```python
from build123d import *

# Parameters (mm, degrees)
SKETCH1_W                          = 165.1
SKETCH1_H                          = 12.7
BOSS_EXTRUDE1_DEPTH                = 127
SKETCH2_R                          = 20.6375
CUT_EXTRUDE1_DEPTH                 = 153.002606886
CUT_EXTRUDE3_DEPTH                 = 153.002606886
FILLET1_R                          = 3.175
FILLET2_R                          = 1.5875
SKETCH5_W                          = 101.6
SKETCH5_H                          = 9.525
CUT_EXTRUDE4_DEPTH                 = 153.002606886
FILLET3_R                          = 3.175
F_1_16_0_0625_DIAMETER_HOLE1_D     = 1.5875
F_1_16_0_0625_DIAMETER_HOLE1_DEPTH = 15.875
F_1_16_0_0625_DIAMETER_HOLE1_TIP   = 0.476933116
F_1_16_0_0625_DIAMETER_HOLE2_D     = 1.5875
F_1_16_0_0625_DIAMETER_HOLE2_DEPTH = 15.875
F_1_16_0_0625_DIAMETER_HOLE2_TIP   = 0.476933116
CUT_EXTRUDE5_DEPTH                 = 153.002606886


with BuildPart() as part:
    # Sketch1 → Boss-Extrude1 (new, symmetric)
    with BuildSketch(Plane(origin=(0, 0, 0), x_dir=(1, 0, 0), z_dir=(0, 1, 0))):
        Rectangle(SKETCH1_W, SKETCH1_H)
    extrude(amount=BOSS_EXTRUDE1_DEPTH, both=True)

    # Sketch2 → Cut-Extrude1 (cut, through all)
    with BuildSketch(Plane.XY.offset(6.35)):
        with Locations((0, 127)):
            Circle(SKETCH2_R)
    extrude(amount=-CUT_EXTRUDE1_DEPTH, mode=Mode.SUBTRACT)

    # Sketch4 → Cut-Extrude3 (cut, through all)
    with BuildSketch(Plane.XY.offset(6.35)):
        with BuildLine():
            Line((57.277, 127), (57.277, 104.775))
            Line((57.277, 104.775), (43.877983689, 104.775))
            Line((43.877983689, 104.775), (38.415383769, 114.236500603))
            ThreePointArc((38.415383769, 114.236500603), (39.624000301, 118.747116057), (44.134615883, 117.5385))
            Line((44.134615883, 117.5385), (47.690804866, 111.379))
            Line((47.690804866, 111.379), (50.673, 111.379))
            Line((50.673, 111.379), (50.673, 127))
            Line((50.673, 127), (57.277, 127))
        make_face()
        with BuildLine():
            Line((-50.673, 127), (-57.277, 127))
            Line((-57.277, 127), (-57.277, 104.775))
            Line((-57.277, 104.775), (-43.877983689, 104.775))
            Line((-43.877983689, 104.775), (-38.415383769, 114.236500603))
            ThreePointArc((-38.415383769, 114.236500603), (-39.624000301, 118.747116057), (-44.134615883, 117.5385))
            Line((-44.134615883, 117.5385), (-47.690804866, 111.379))
            Line((-47.690804866, 111.379), (-50.673, 111.379))
            Line((-50.673, 111.379), (-50.673, 127))
        make_face()
    extrude(amount=-CUT_EXTRUDE3_DEPTH, mode=Mode.SUBTRACT)

    # Fillet1
    fillet1_edges = [part.edges().sort_by_distance(p)[0] for p in [
        (50.673, 127, 0),
        (57.277, 127, 0),
        (57.277, 104.775, 0),
        (43.877983689, 104.775, 0),
        (-43.877983689, 104.775, 0),
        (-57.277, 104.775, 0),
        (-57.277, 127, 0),
        (-50.673, 127, 0),
    ]]
    fillet(fillet1_edges, radius=FILLET1_R)

    # Fillet2
    fillet2_edges = [part.edges().sort_by_distance(p)[0] for p in [
        (47.690804866, 111.379, 0),
        (50.673, 111.379, 0),
        (-50.673, 111.379, 0),
        (-47.690804866, 111.379, 0),
    ]]
    fillet(fillet2_edges, radius=FILLET2_R)

    # Sketch5 → Cut-Extrude4 (cut, through all)
    with BuildSketch(Plane.XY.offset(6.35)):
        with Locations((0, -122.2375)):
            Rectangle(SKETCH5_W, SKETCH5_H)
    extrude(amount=-CUT_EXTRUDE4_DEPTH, mode=Mode.SUBTRACT)

    # Fillet3
    fillet3_edges = [part.edges().sort_by_distance(p)[0] for p in [
        (-50.8, -127, 0),
        (-50.8, -117.475, 0),
        (50.8, -117.475, 0),
        (50.8, -127, 0),
    ]]
    fillet(fillet3_edges, radius=FILLET3_R)

    # 1/16 (0.0625) Diameter Hole1
    with Locations(Plane(origin=(82.55, 0, 0), x_dir=(0, 0, -1), z_dir=(1, 0, 0))):
        with Locations((0, -120.65), (0, -95.25), (0, 44.45), (0, 69.85), (0, 120.65)):
            Hole(F_1_16_0_0625_DIAMETER_HOLE1_D / 2, depth=F_1_16_0_0625_DIAMETER_HOLE1_DEPTH)
            with Locations((0, 0, -(F_1_16_0_0625_DIAMETER_HOLE1_DEPTH + F_1_16_0_0625_DIAMETER_HOLE1_TIP / 2))):  # 118° drill point
                Cone(0, F_1_16_0_0625_DIAMETER_HOLE1_D / 2, F_1_16_0_0625_DIAMETER_HOLE1_TIP, mode=Mode.SUBTRACT)

    # 1/16 (0.0625) Diameter Hole2
    with Locations(Plane.ZY.offset(82.55)):
        with Locations((0, -120.65), (0, -95.25), (0, 44.45), (0, 69.85), (0, 120.65)):
            Hole(F_1_16_0_0625_DIAMETER_HOLE2_D / 2, depth=F_1_16_0_0625_DIAMETER_HOLE2_DEPTH)
            with Locations((0, 0, -(F_1_16_0_0625_DIAMETER_HOLE2_DEPTH + F_1_16_0_0625_DIAMETER_HOLE2_TIP / 2))):  # 118° drill point
                Cone(0, F_1_16_0_0625_DIAMETER_HOLE2_D / 2, F_1_16_0_0625_DIAMETER_HOLE2_TIP, mode=Mode.SUBTRACT)

    # Sketch10 → Cut-Extrude5 (cut, through all)
    with BuildSketch(Plane.XY.offset(6.35)):
        with BuildLine():
            Line((-61.89437725, -88.484920775), (-50.783316982, 38.515079225))
            ThreePointArc((-50.783316982, 38.515079225), (-45.623860507, 42.84437725), (-41.294562483, 37.684920775))
            Line((-41.294562483, 37.684920775), (-52.40562275, -89.315079225))
            ThreePointArc((-52.40562275, -89.315079225), (-57.565079225, -93.64437725), (-61.89437725, -88.484920775))
        make_face()
        with BuildLine():
            Line((-27.00562275, -89.315079225), (-15.894562483, 37.684920775))
            ThreePointArc((-15.894562483, 37.684920775), (-20.223860507, 42.84437725), (-25.383316982, 38.515079225))
            Line((-25.383316982, 38.515079225), (-36.49437725, -88.484920775))
            ThreePointArc((-36.49437725, -88.484920775), (-32.165079225, -93.64437725), (-27.00562275, -89.315079225))
        make_face()
        with BuildLine():
            Line((-1.60562275, -89.315079225), (9.505437517, 37.684920775))
            ThreePointArc((9.505437517, 37.684920775), (5.176139493, 42.84437725), (0.016683018, 38.515079225))
            Line((0.016683018, 38.515079225), (-11.09437725, -88.484920775))
            ThreePointArc((-11.09437725, -88.484920775), (-6.765079225, -93.64437725), (-1.60562275, -89.315079225))
        make_face()
        with BuildLine():
            Line((23.79437725, -89.315079225), (34.905437517, 37.684920775))
            ThreePointArc((34.905437517, 37.684920775), (30.576139493, 42.84437725), (25.416683018, 38.515079225))
            Line((25.416683018, 38.515079225), (14.30562275, -88.484920775))
            ThreePointArc((14.30562275, -88.484920775), (18.634920775, -93.64437725), (23.79437725, -89.315079225))
        make_face()
        with BuildLine():
            Line((49.19437725, -89.315079225), (60.305437517, 37.684920775))
            ThreePointArc((60.305437517, 37.684920775), (55.976139493, 42.84437725), (50.816683018, 38.515079225))
            Line((50.816683018, 38.515079225), (39.70562275, -88.484920775))
            ThreePointArc((39.70562275, -88.484920775), (44.034920775, -93.64437725), (49.19437725, -89.315079225))
        make_face()
    extrude(amount=-CUT_EXTRUDE5_DEPTH, mode=Mode.SUBTRACT)


solid = part.part
```
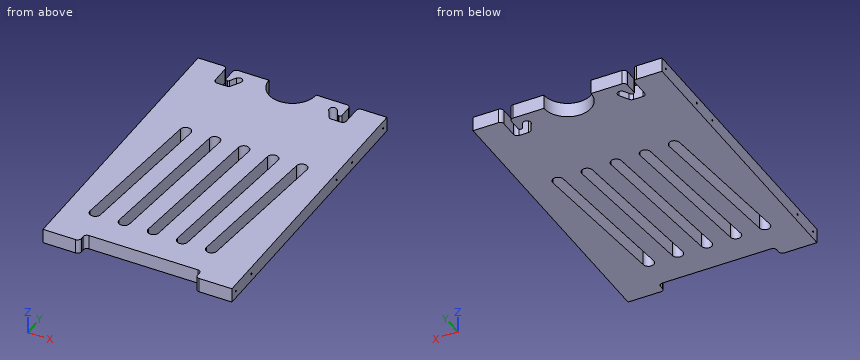
Read the model definition and answer for the solid it produces. Units are mm, in the model's axes. Coordinates: 2 decimals unless noted, no trailing zeros. Loops run counter-clockwise (first coordinate to the right, second up) from the corner with the lowest first, then second, coordinate; pieces in that order, holes last.
(1) The part is cut by section C-C (z = 3). Count the separate pieces of the cut face and the enclosed holes in it, and give its area (3 significant figures).
Solution:
separate pieces: 1
enclosed holes: 5
area: 33,400 mm2
(2) Consider line 1 along Y through (x, z) = (-76.5, 0); line 2 along X through (y, z) = (-23, -0.5); line 3 along X through (y, z) = (-89.5, 1). Determine where each line is inside the solid, lowest interval first.
Solution:
line 1: y = -127 to -121.44, -119.86 to -96.04, -94.46 to 43.66, 45.24 to 69.06, 70.64 to 119.86, 121.44 to 127
line 2: x = -82.55 to -56.17, -46.6 to -30.77, -21.2 to -5.37, 4.2 to 20.03, 29.6 to 45.43, 55 to 82.55
line 3: x = -82.55 to -61.87, -52.43 to -36.47, -27.03 to -11.07, -1.63 to 14.33, 23.77 to 39.73, 49.17 to 82.55
(3) The part is cut by section A-A (y = -27). Determine the outline of the cut face in (x, z), and give its area (3 significant figures).
Solution:
outline: (-82.55, -6.35) - (-56.52, -6.35) - (-56.52, 6.35) - (-82.55, 6.35) - close; (-46.95, -6.35) - (-31.12, -6.35) - (-31.12, 6.35) - (-46.95, 6.35) - close; (-21.55, -6.35) - (-5.72, -6.35) - (-5.72, 6.35) - (-21.55, 6.35) - close; (3.85, -6.35) - (19.68, -6.35) - (19.68, 6.35) - (3.85, 6.35) - close; (29.25, -6.35) - (45.08, -6.35) - (45.08, 6.35) - (29.25, 6.35) - close; (54.65, -6.35) - (82.55, -6.35) - (82.55, 6.35) - (54.65, 6.35) - close
area: 1,490 mm2
(4) Flat-ended cylindrical pins translate along their axes: pin 1 Ø1.3 at (y, z) = (120.65, 0) entering from -X; pin 2 Ø1 at (x, z) = (-6, 2.5) entering from -Y (3 decimals). Find the tip coordinate at first contact, or state that the pin passes through.
Solution:
pin 1: stops at x = -66.59
pin 2: stops at y = -117.475
